Autodesk Inventor part; units mm, degrees
ref_plane "YZ Plane" through (0, 0, 0) normal (1, 0, 0) x (0, 1, 0)
ref_plane "XZ Plane" through (0, 0, 0) normal (0, 1, 0) x (-1, 0, 0)
ref_plane "XY Plane" through (0, 0, 0) normal (0, 0, 1) x (1, 0, 0)
sketch "Sketch1" plane through (0, 0, 0) normal (0, 0, 1) x (1, 0, 0)
  circle A0 centre (0, 0) radius 3.925
  circle A1 centre (0, 0) radius 2.286
  dimension "d0" = 7.85
  dimension "d1" = 4.572
extrude "Extrusion1" add sketch "Sketch1" against normal blind 7
sketch "Sketch2" plane through (0, 0, -7) normal (0, 0, -1) x (-1, 0, 0)
  circle A0 centre (0, 0) radius 6.05
  circle A1 centre (0, 0) radius 2.286
  dimension "d4" = 12.1
extrude "Extrusion2" add sketch "Sketch2" along normal blind 1.27
chamfer "Chamfer1" distance 0.6 angle 45 1 edges at (2.286, 0, -8.27)
properties part number "bearingsleeve_3DPrint"
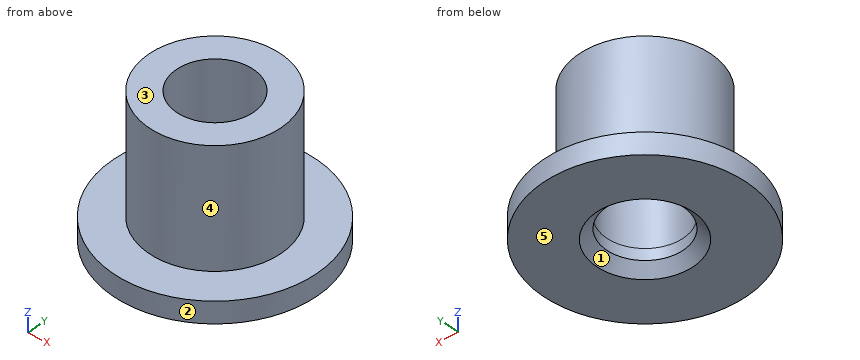
The model under review builds one solid part; all positions refer to its coordinate system, in mm. Face numbers are marked on the shaded views. A direction names the side the tool comes from. Round coordinates to 2 decimals unless told otherwise and drop trailing zeros. Loops run counter-clockwise (first coordinate to the right, second up) from the corner with the lowest first, then second, coordinate; pieces in that order, holes last. Notation, with made-up numbers: (71, 77) -> (122, 77) arc R33 ccw to (122, 106) -> close; hole circle Ø11 at (-2.75, 9.25). An arc over 180 degrees is marked (long way). Return JSON: item names as keys, results as strings.
(1) The part is to be moulded in two halves that separate along X. For the marked faces 1, 2 and 3, say which applies: released by +X, released by -X, zero draft, split by the parting line, or undercut.
Solved:
{"face 1": "undercut", "face 2": "split by the parting line", "face 3": "zero draft"}
(2) For the marked faces 4 and 5, list the 3-axis set-ups (+Z, -Z, +X, -X, +Y, -Y) from which the entire face can be reached by the end or side of a thin tool; tool diameter is ignored.
Solved:
{"face 4": "+Z", "face 5": "-Z, +X, -X, +Y, -Y"}
(3) For pin 1 (1 mm diameter, centred on x = 0, y = 2, fed in from -Z); pin 2 (1.5 mm diameter, centred on x = -1.5, z = -4, fed in from -Y); pin 3 (1 mm diameter, centred on x = -4.5, z = -5.5, fed in from +Y); pin 4 (6 mm diameter, centred on x = 0, y = 0, fed in from -Z), all flat-tipped, find the tip position at first contact; note any pin that passes through.
Solved:
{"pin 1": "z = -7.88", "pin 2": "y = -3.85", "pin 3": "through", "pin 4": "z = -8.27"}
(4) Add section A-A on x = 0. Write out the cut boundary in (y, z) (3 decimals).
Solved:
{"outline": "(-6.05, -8.27) -> (-2.886, -8.27) -> (-2.286, -7.67) -> (-2.286, 0) -> (-3.925, 0) -> (-3.925, -7) -> (-6.05, -7) -> close; (2.286, -7.67) -> (2.886, -8.27) -> (6.05, -8.27) -> (6.05, -7) -> (3.925, -7) -> (3.925, 0) -> (2.286, 0) -> close"}
(5) Add section C-C on z = -5.5. Write out the cut boundary in (x, y) (3 decimals), plus the area to 3 significant figures.
Solved:
{"outline": "circle Ø7.85 at (0, 0); hole circle Ø4.572 at (0, 0)", "area": "32.0 mm2"}
(6) Add section D-D on x = 3.5. Write out the cut boundary in (y, z), plus the area to 3 significant figures.
Solved:
{"outline": "(-4.93, -8.27) -> (4.93, -8.27) -> (4.93, -7) -> (1.78, -7) -> (1.78, 0) -> (-1.78, 0) -> (-1.78, -7) -> (-4.93, -7) -> close", "area": "37.4 mm2"}
(7) For line 1 (Y direction, x = 0, z = -7.5); line 2 (Z direction, x = -1.5, y = -4.75); line 3 (Y direction, x = 0.75, z = -1.25), list the stretches that pass through material, from the lowest coordinate up.
Solved:
{"line 1": "-6.05 to -2.29, 2.29 to 6.05", "line 2": "-8.27 to -7", "line 3": "-3.85 to -2.16, 2.16 to 3.85"}
